Source: CAD feature listing. Evaluate the final solid. Frame: model axes, mm. Face numbers are marked on the shaded views. A direction names the side the tool comes from. Give positions to 0.01 mm unless a question says otherwise; leave off trailing zeros. Write each loop counter-clockwise with the first axis right and the second up, starting at its lowest first coordinate (ties: lowest second). Pieces come first, ordered by that corner, then holes. Notation, with made-up numbers: M -23.5,-31 L -0.5,-31 A16 ccw -0.5,-2 Z; hole C 11.5,-35 d3. An arc over 180 degrees is marked long. Return JSON: item names as keys, results as strings.
```python
from build123d import *

# Parameters (mm, degrees)
PAD_DEPTH      = 200
PAD001_DEPTH   = 10
PAD002_DEPTH   = 50
SKETCH003_R    = 3
HOLE_DEPTH     = 25
HOLE_TIPS_R    = 3
SKETCH004_R    = 3
HOLE001_DEPTH  = 25
HOLE001_TIPS_R = 3


with BuildPart() as part:
    # Sketch → Pad (new body)
    with BuildSketch(Plane.XZ):
        with BuildLine():
            Line((-32, 32), (32, 32))
            ThreePointArc((28, 28), (30.828427, 29.171573), (32, 32))
            Line((4, 28), (28, 28))
            Line((4, 28), (4, 4))
            ThreePointArc((-4, 4), (0, 0), (4, 4))
            Line((-4, 4), (-4, 28))
            Line((-28, 28), (-4, 28))
            ThreePointArc((-32, 32), (-30.828427, 29.171573), (-28, 28))
        make_face()
    extrude(amount=PAD_DEPTH)

    # Sketch001 (on DatumPlane) → Pad001 (join, symmetric)
    with BuildSketch(Plane(origin=(0, 0, 0), x_dir=(0, -1, 0), z_dir=(1, 0, 0))):
        with BuildLine():
            Line((200, 0), (232, 0))
            ThreePointArc((228, -4), (230.828427, -2.828427), (232, 0))
            Line((228, -4), (204, -4))
            Line((204, -4), (204, -28))
            ThreePointArc((200, -32), (202.828427, -30.828427), (204, -28))
            Line((200, 0), (200, -32))
        make_face()
    extrude(amount=PAD001_DEPTH, both=True)

    # Sketch002 (on DatumPlane) → Pad002 (join, symmetric)
    with BuildSketch(Plane(origin=(0, 0, 0), x_dir=(0, -1, 0), z_dir=(1, 0, 0))):
        with BuildLine():
            Line((0, 0), (-32, 0))
            ThreePointArc((-32, 0), (-30.828427, -2.828427), (-28, -4))
            Line((-28, -4), (-4, -4))
            Line((-4, -4), (-4, -28))
            ThreePointArc((-4, -28), (-2.828427, -30.828427), (0, -32))
            Line((0, 0), (0, -32))
        make_face()
    extrude(amount=PAD002_DEPTH, both=True)

    # Sketch003 (on Face22 of Pad002) → Hole (cut)
    with BuildSketch(Plane(origin=(0, 0, 0), x_dir=(1, 0, 0), z_dir=(0, 0, -1))):
        with Locations((0, 216)):
            Circle(SKETCH003_R)
    extrude(amount=-HOLE_DEPTH, mode=Mode.SUBTRACT)

    # Hole tips → Hole tip 1 section 0
    with BuildSketch(Plane(origin=(0, 0, 25), x_dir=(1, 0, 0), z_dir=(0, 0, -1)), mode=Mode.PRIVATE) as hole_tip_1_s0:
        with Locations((0, 216)):
            Circle(HOLE_TIPS_R)
    loft([hole_tip_1_s0.sketch, Vertex(0, -216, 26.802582)], mode=Mode.SUBTRACT)

    # Sketch004 (on Face14 of Hole) → Hole001 (cut)
    with BuildSketch(Plane(origin=(0, 0, 0), x_dir=(1, 0, 0), z_dir=(0, 0, -1))):
        with Locations((34, -16)):
            Circle(SKETCH004_R)
        with Locations((-34, -16)):
            Circle(SKETCH004_R)
    extrude(amount=-HOLE001_DEPTH, mode=Mode.SUBTRACT)

    # Hole001 tips → Hole001 tip 1 section 0
    with BuildSketch(Plane(origin=(0, 0, 25), x_dir=(1, 0, 0), z_dir=(0, 0, -1)), mode=Mode.PRIVATE) as hole001_tip_1_s0:
        with Locations((34, -16)):
            Circle(HOLE001_TIPS_R)
    loft([hole001_tip_1_s0.sketch, Vertex(34, 16, 26.802582)], mode=Mode.SUBTRACT)

    # Hole001 tips → Hole001 tip 2 section 0
    with BuildSketch(Plane(origin=(0, 0, 25), x_dir=(1, 0, 0), z_dir=(0, 0, -1)), mode=Mode.PRIVATE) as hole001_tip_2_s0:
        with Locations((-34, -16)):
            Circle(HOLE001_TIPS_R)
    loft([hole001_tip_2_s0.sketch, Vertex(-34, 16, 26.802582)], mode=Mode.SUBTRACT)


solid = part.part
```
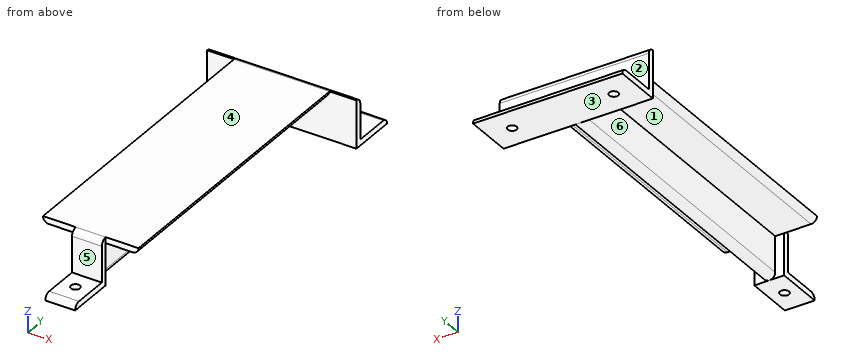
1) Line query: line 1 (X direction, y = 16, z = 3.2); line 2 (X direction, y = -216, z = 1); line 3 (Y direction, x = 6, z = 18). Output: solid intervals per line, ascending. Write a range as [from, to].
Numbers:
{"line 1": "x = [-50, -37], [-31, 31], [37, 50]", "line 2": "x = [-10, -3], [3, 10]", "line 3": "y = [-204, -200], [0, 4]"}
2) Cut plane D-D, the plane x = -42. Return the cut outline in (y, z).
Numbers:
{"outline": "M 0,0 L 32,0 A4 ccw 28,4 L 4,4 L 4,28 A4 ccw 0,32 Z"}
3) Set-up query: the marked faces 4, 5 and 6. Return all of +Z, -Z, +X, -X, +Y, -Y with unobstructed straight access to the full face (end or side cutting, diameter ignored); none if empty.
Numbers:
{"face 4": "+Z, +X, -X, +Y, -Y", "face 5": "+Z, +X, -X, -Y", "face 6": "-Z, -X"}
4) Cut plane A-A, the plane y = 16. Return the cut outline in (x, z).
Numbers:
{"outline": "M -50,0 L -37,0 L -37,4 L -50,4 Z; M -31,0 L 31,0 L 31,4 L -31,4 Z; M 37,0 L 50,0 L 50,4 L 37,4 Z"}
5) Contact query for flat-ended pins moving along their axis: pin 1 Ø6 at (x, y) = (-2.5, -214.5) entering from +Z; pin 2 Ø11 at (x, z) = (5.5, 18.5) entering from +Y; pin 3 Ø1.5 at (y, z) = (-200, 19) entering from -X; pin 4 Ø12 at (x, y) = (1, -185) entering from -Z. Output: stop coordinate, or through.
Numbers:
{"pin 1": "stops at z = 4", "pin 2": "stops at y = 4", "pin 3": "stops at x = -10", "pin 4": "stops at z = 0"}
6) Cut plane B-B, the plane y = -115. Return the cut outline in (x, z), then the cut area to 3 significant figures.
Numbers:
{"outline": "M -32,32 A4 ccw -28,28 L -4,28 L -4,4 A4 ccw 4,4 L 4,28 L 28,28 A4 ccw 32,32 Z", "area": "466 mm²"}
7) Draft query along Y for the marked faces 1, 2 and 3. Return one class per face: released by +Y, released by -Y, zero draft, split by the parting line, or undercut.
Numbers:
{"face 1": "undercut", "face 2": "released by +Y", "face 3": "zero draft"}
8) Cut plane C-C, the plane z = 22. Return the cut outline in (x, y).
Numbers:
{"outline": "M -50,0 L -4,0 L -4,-200 L -10,-200 L -10,-204 L 10,-204 L 10,-200 L 4,-200 L 4,0 L 50,0 L 50,4 L -50,4 Z"}
